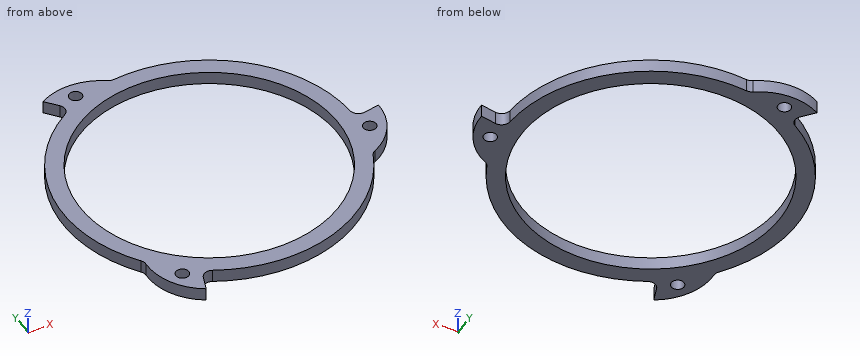
Autodesk Inventor part; units mm, degrees
ref_plane "YZ Plane" through (0, 0, 0) normal (1, 0, 0) x (0, 1, 0)
ref_plane "XZ Plane" through (0, 0, 0) normal (0, 1, 0) x (-1, 0, 0)
ref_plane "XY Plane" through (0, 0, 0) normal (0, 0, 1) x (1, 0, 0)
sketch "Sketch1" plane through (0, 0, 0) normal (0, 0, 1) x (1, 0, 0)
  circle A0 centre (0, 0) radius 63.5 construction
  circle A1 centre (0, 0) radius 47.625
  circle A2 centre (0, 0) radius 53.975
  line L0 (0, 0) -> (63.5, 0) construction
  line L1 (63.5, 0) -> (53.948719, -1.684149)
  arc A3 (49.945192, -20.464076) -> (63.5, 0) centre (41.275, 0) ccw
  line L2 (-31.75, 54.992613) -> (-25.515844, 47.563035)
  arc A4 (-7.250187, 53.485843) -> (-31.75, 54.992613) centre (-20.6375, 35.745199) ccw
  line L3 (-31.75, -54.992613) -> (-28.432875, -45.878887)
  arc A5 (-42.695005, -33.021768) -> (-31.75, -54.992613) centre (-20.6375, -35.745199) ccw
  circle A6 centre (25.4, 0) radius 22.225
  circle A7 centre (-11.250284, 22.225) radius 20.6375
  circle A8 centre (-11.250284, 22.225) radius 7.9375
  circle A9 centre (-39.6875, 0) radius 7.9375
  circle A10 centre (19.84375, -34.370383) radius 7.9375
  circle A11 centre (19.84375, 34.370383) radius 7.9375
  circle A12 centre (25.4, 0) radius 2
  circle A13 centre (-11.250284, -22.225) radius 20.6375
  circle A14 centre (-11.250284, -22.225) radius 7.9375
  circle A15 centre (55.794471, -7.9375) radius 2.38125
  circle A16 centre (-21.023159, 52.288179) radius 2.38125
  circle A17 centre (-34.771312, -44.350679) radius 2.38125
  point P0 (-7.250187, 53.485843)
  point P1 (-25.515844, 47.563035)
  point P2 (-42.695005, -33.021768)
  point P3 (-28.432875, -45.878887)
  dimension "Ring_OD" = 127
  dimension "d2" = 6.35
  dimension "d3" = 9.525
  dimension "d15" = 10
  dimension "d16" = 22.225
  dimension "d19" = 360
  dimension "Pulley_OD" = 44.45
  dimension "Brass_OD" = 41.275
  dimension "d41" = 15.875
  dimension "Brass_Offset" = 22.225
  dimension "d43" = 15.875
  dimension "d46" = 360
  dimension "d48" = 4
  dimension "d50" = 4.7625
  dimension "d51" = 7.9375
  dimension "d54" = 360
  dimension "Ring_ID" = 95.25
sketch "Sketch1 outline for Extrusion1" plane through (0, 0, 0) normal (0, 0, 1) x (1, 0, 0)
  arc A0 (49.945192, -20.464076) -> (63.5, 0) centre (41.275, 0) ccw
  arc A1 (-28.432875, -45.878887) -> (49.945192, -20.464076) centre (0, 0) ccw
  line L0 (63.5, 0) -> (53.948719, -1.684149)
  line L1 (-31.75, -54.992613) -> (-28.432875, -45.878887)
  arc A2 (53.948719, -1.684149) -> (-7.250187, 53.485843) centre (0, 0) ccw
  arc A3 (-42.695005, -33.021768) -> (-31.75, -54.992613) centre (-20.6375, -35.745199) ccw
  arc A4 (-7.250187, 53.485843) -> (-31.75, 54.992613) centre (-20.6375, 35.745199) ccw
  arc A5 (-25.515844, 47.563035) -> (-42.695005, -33.021768) centre (0, 0) ccw
  line L2 (-31.75, 54.992613) -> (-25.515844, 47.563035)
  circle A6 centre (-34.771312, -44.350679) radius 2.38125
  circle A7 centre (0, 0) radius 47.625
  circle A8 centre (55.794471, -7.9375) radius 2.38125
  circle A9 centre (-21.023159, 52.288179) radius 2.38125
extrude "Extrusion1" add sketch "Sketch1 outline for Extrusion1" along normal blind 4.7625
fillet "Fillet1" radius 3.175 6 edges at (-7.2502, 53.4858, 2.3813) (-25.5158, 47.563, 2.3813) (53.9487, -1.6841, 2.3813) (49.9452, -20.4641, 2.3813) (-28.4329, -45.8789, 2.3813) (-42.695, -33.0218, 2.3813)
properties part number "Ring Vert Test" material "Steel, Alloy"
The listing builds one solid part. Answer for the finished solid, in the listing's coordinates (mm). Give positions to 0.01 mm unless a question says otherwise; leave off trailing zeros. Loops run counter-clockwise (first coordinate to the right, second up) from the corner with the lowest first, then second, coordinate; pieces in that order, holes last.
Item 1: A cutting plane is placed at B-B (y = 23). Give the vertices of the cut face in (x, z).
Derived:
outline: (-48.83, 0) - (-41.7, 0) - (-41.7, 4.76) - (-48.83, 4.76) - close; (41.7, 0) - (48.83, 0) - (48.83, 4.76) - (41.7, 4.76) - close
Item 2: This flat-tipped pin is pushed along its axis until it touches: pin 1 Ø1 at (y, z) = (41, 2.5) entering from +X. Where does it stop, or does it pass through?
Derived:
pin 1: stops at x = 35.68
Item 3: Find the intervals of material crossed by line 1 along X through (y, z) = (34, 3.7); line 2 along X through (y, z) = (26, 1.8); line 3 along Y through (x, z) = (-7, 0.65), in increasing order.
Derived:
line 1: x = -41.92 to -33.35, 33.35 to 41.92
line 2: x = -47.3 to -39.9, 39.9 to 47.3
line 3: y = -53.52 to -47.11, 47.11 to 53.67
Item 4: A cutting plane is placed at A-A (x = 0). Give the vertices of the cut face in (y, z) (1 decimal).
Derived:
outline: (-54, 0) - (-47.6, 0) - (-47.6, 4.8) - (-54, 4.8) - close; (47.6, 0) - (54, 0) - (54, 4.8) - (47.6, 4.8) - close
